from build123d import *

# Parameters (mm, degrees)
F1_DEPTH = 6


with BuildPart() as f1:
    # F0 (on Front) → F1 (new body, symmetric)
    with BuildSketch(Plane.XZ):
        Polygon((-395.130562, -79.500396), (-395.130562, -240.300396), (209.869438, -240.300396), (209.869438, -160.300396), (264.869438, -160.300396), (264.869438, 259.699604), (324.869438, 259.699604), (324.869438, 299.699604), (304.869438, 299.699604), (304.869438, 280.499604), (224.069438, 280.499604), (224.069438, 230.499604), (204.869438, 230.499604), (204.869438, 280.499604), (104.869438, 280.499604), (104.869438, 299.699604), (84.869438, 299.699604), (84.869438, 119.699604), (134.869438, 119.699604), (134.869438, 100.499604), (-25.930562, 100.499604), (-25.930562, 50.499604), (-45.130562, 50.499604), (-45.130562, 100.499604), (-155.130562, 100.499604), (-155.130562, -60.300396), (-105.130562, -60.300396), (-105.130562, -79.500396), (-172.839355, -79.500396), (-265.930562, -79.500396), (-265.930562, -129.500396), (-285.130562, -129.500396), (-285.130562, -79.500396), align=None)
    extrude(amount=F1_DEPTH, both=True)


solid = f1.part
The model under review builds one solid part; all positions refer to its coordinate system, in mm. Round coordinates to 2 decimals unless told otherwise and drop trailing zeros. Order: outer loops, then holes, each group sorted by start corner. A loop starts at its lowest first (then second) coordinate and runs counter-clockwise, first axis right, second up. Notation, with made-up numbers: (17.5, 34.5) -> (72.5, 34.5) arc R14 cw to (72.5, 48.5) -> close; hole circle Ø1 at (57, -30.5). An arc over 180 degrees is marked (long way). Write item = value, one per line. Start each with the question number.
Item 1: Consider section B-B on x = -91.5. Write out the cut boundary in (y, z).
Item 2: For line 1 along X through (y, z) = (-5.5, -95); line 2 along X through (y, z) = (-5.25, 273.5); line 3 along Z through (x, y) = (-336.5, -0.25), list the stretches that pass through material, from the lowest coordinate up.
Item 3: Consider section C-C on z = -187. Write out the cut boundary in (x, y), plus the area to 3 significant figures.
Item 4: Clearance check with flat-ended pins moving along their axes: pin 1 Ø6 at (y, z) = (1, 206) entering from -X; pin 2 Ø2 at (y, z) = (-4.5, -41) entering from -X; pin 3 Ø3.5 at (x, y) = (-172, -1.5) entering from +Z. State where each tip first meets the part, or that it passes through.
Conclusion:
q1.outline = (-6, -240.3) -> (6, -240.3) -> (6, 100.5) -> (-6, 100.5) -> close
q2.line_1 = -395.13 to -285.13, -265.93 to 264.87
q2.line_2 = 84.87 to 204.87, 224.07 to 324.87
q2.line_3 = -240.3 to -79.5
q3.outline = (-395.13, -6) -> (209.87, -6) -> (209.87, 6) -> (-395.13, 6) -> close
q3.area = 7,260 mm2
q4.pin_1 = 84.87
q4.pin_2 = -155.13
q4.pin_3 = -79.5
